Verification items for this drawing (mm, ordinates from the low corner). Give positions to 0.01 mm unless a question says otherwise; leave off trailing zeros. Order: outer loops, then holes, each group sorted by start corner. A loop starts at its lowest first (then second) coordinate and runs counter-clockwise, first axis right, second up.
(1) Sectioned sample at A-A on z = 19.05. Record the cut outline in (x, y).
(2) Mould release check, pull along X, two halves, no side actions. Record for the marked faces 1, 2 and 3: pulls with the +X half, pulls with the -X half, needs draft (parallel to the pull), parting line crosses it, or undercut.
(3) Sectioned sample at D-D on z = 26.5. Record the cut outline in (x, y), plus the area to 3 significant figures.
(4) Scan lines: L1, parallel to X at y = 6.75, z = 19.5; L2, parallel to X at y = 2, z = 7.5; L3, parallel to Z at x = 171.45, y = 6. Record each from-to range of solid material in increasing order.
(5) Sectioned sample at C-C on y = 2.5. Record the cut outline in (x, z).
(6) Sectioned sample at B-B on x = 19.05. Record the cut outline in (y, z).
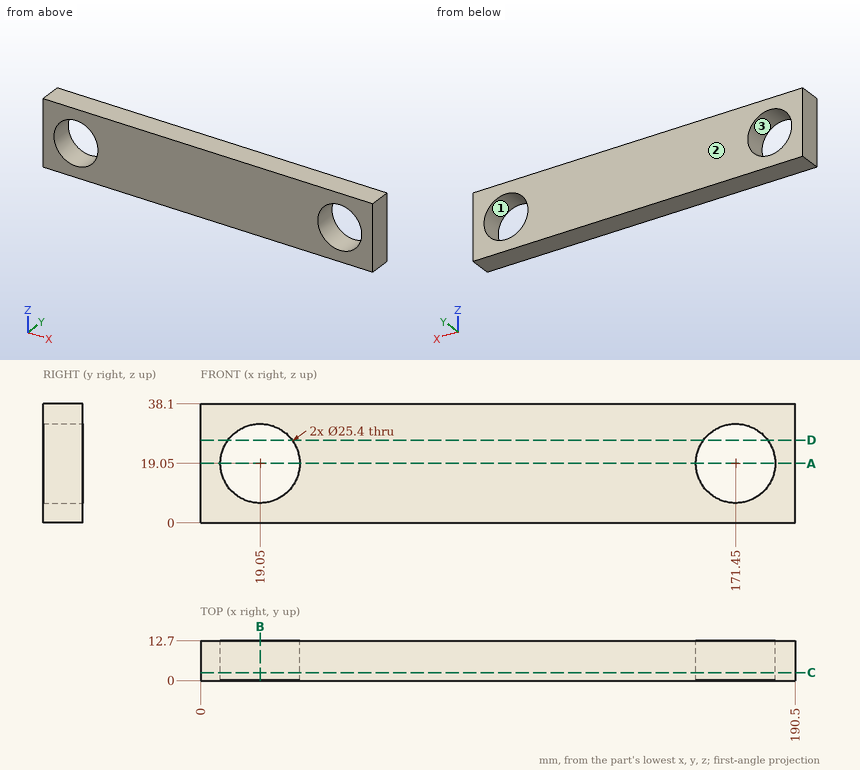
Ans:
1. outline: (0, 0) - (6.35, 0) - (6.35, 12.7) - (0, 12.7) - close; (31.75, 0) - (158.75, 0) - (158.75, 12.7) - (31.75, 12.7) - close; (184.15, 0) - (190.5, 0) - (190.5, 12.7) - (184.15, 12.7) - close
2. face 1: undercut
2. face 2: needs draft
2. face 3: undercut
3. outline: (0, 0) - (8.76, 0) - (8.76, 12.7) - (0, 12.7) - close; (29.34, 0) - (161.16, 0) - (161.16, 12.7) - (29.34, 12.7) - close; (181.74, 0) - (190.5, 0) - (190.5, 12.7) - (181.74, 12.7) - close
3. area: 1,900 mm2
4. L1: x = 0 to 6.36, 31.74 to 158.76, 184.14 to 190.5
4. L2: x = 0 to 13.77, 24.33 to 166.17, 176.73 to 190.5
4. L3: z = 0 to 6.35, 31.75 to 38.1
5. outline: (0, 0) - (190.5, 0) - (190.5, 38.1) - (0, 38.1) - close; hole circle Ø25.4 at (19.05, 19.05); hole circle Ø25.4 at (171.45, 19.05)
6. outline: (0, 0) - (12.7, 0) - (12.7, 6.35) - (0, 6.35) - close; (0, 31.75) - (12.7, 31.75) - (12.7, 38.1) - (0, 38.1) - close
